Read the model definition and answer for the solid it produces. Units are mm, in the model's axes. A direction names the side the tool comes from. Coordinates: 2 decimals unless noted, no trailing zeros. Order: outer loops, then holes, each group sorted by start corner. A loop starts at its lowest first (then second) coordinate and runs counter-clockwise, first axis right, second up. Notation, with made-up numbers: M -0.5,-21 L 20.5,-21 A11 ccw 20.5,0 Z; hole C 50.25,-29 d5. An arc over 180 degrees is marked long. Write each question's results on one line, items separated by ' | '.
Autodesk Inventor part; units mm, degrees
ref_plane "YZ Plane" through (0, 0, 0) normal (1, 0, 0) x (0, 1, 0)
ref_plane "XZ Plane" through (0, 0, 0) normal (0, 1, 0) x (-1, 0, 0)
ref_plane "XY Plane" through (0, 0, 0) normal (0, 0, 1) x (1, 0, 0)
sketch "Sketch1" plane through (0, 0, 0) normal (0, 0, 1) x (1, 0, 0)
  circle A0 centre (0, 0) radius 1.5
  circle A1 centre (0, 30.5) radius 1.5
  line L0 (0, 8.5) -> (-4, 4.5)
  line L1 (-4, 35) -> (-4, 25.5)
  line L2 (-4, 4.5) -> (-4, -5)
  line L3 (0, 21) -> (0, 8.5)
  line L4 (-4, 35) -> (5, 35)
  line L5 (-4, -5) -> (5, -5)
  line L6 (5, 35) -> (5, -5)
  line L7 (0, 21) -> (0, 23.5)
  line L8 (-4, 25.5) -> (-4, 28)
  line L9 (-4, 28) -> (0, 23.5)
  dimension "d0" = 3
  dimension "d1" = 3
  dimension "d47" = 9
  dimension "d48" = 9
  dimension "d52" = 4
  dimension "d55" = 4.5
  dimension "d59" = 40
  dimension "d60" = 2.5
  dimension "d61" = 2.5
extrude "Extrusion1" add sketch "Sketch1" along normal blind 1
fillet "Fillet9" radius 5 2 edges at (5, 35, 0.5) (5, -5, 0.5)
fillet "Fillet10" radius 4 2 edges at (-4, 35, 0.5) (-4, -5, 0.5)
fillet "Fillet11" radius 7.8 2 edges at (0, 8.5, 0.5) (-4, 4.5, 0.5)
fillet "Fillet12" radius 7.8 2 edges at (-4, 28, 0.5) (0, 23.5, 0.5)
properties part number "arm1" material "ABS Plastic"
(1) Straight lines are drawn through the part: line 1 (X direction, y = 14, z = 0.5); line 2 (X direction, y = 1, z = 0.1); line 3 (Y direction, x = 3, z = 0.75). For each, find the intervals that lie inside material, in ascending order.
Conclusion:
line 1: 0 to 5 | line 2: -4 to -1.12, 1.12 to 5 | line 3: -4 to 34
(2) The part is cut by section D-D, the plane x = 2. Write down the section's boundary in (y, z), then the cut area to 3 significant figures.
Conclusion:
outline: M -4.58,0 L 34.58,0 L 34.58,1 L -4.58,1 Z | area: 39.2 mm²
(3) The mould has two halves that part along X. Classify faces 3 (the cylindrical face through (-1.5, -0.07, 0.49)), 4 (the cylindrical face through (-2.797, 33.859, 0.507)), 5 (the cylindrical face through (3.5, -3.57, 0.51)), 6 (the cylindrical face through (-0.195, 29.013, 0.493)): pulls with the +X half, pulls with the -X half, needs draft (parallel to the pull), parting line crosses it, or undercut.
Conclusion:
face 3: undercut | face 4: pulls with the -X half | face 5: pulls with the +X half | face 6: undercut
(4) The part is cut by section A-A, the plane y = 30.5. Write down the section's boundary in (x, z), then the cut area to 3 significant figures.
Conclusion:
outline: M -3.99,0 L -1.5,0 L -1.5,1 L -3.99,1 Z; M 1.5,0 L 4.97,0 L 4.97,1 L 1.5,1 Z | area: 5.96 mm²
(5) For faces 1 (the cylindrical face through (3.57, 33.5, 0.51)), 2 (the cylindrical face through (-3.505, 28.231, 0.507)), determine the directions among +Z, -Z, +X, -X, +Y, -Y from which every point of the face is accessible in a straight line to the end or side of a thin tool.
Conclusion:
face 1: +Z, -Z, +X, +Y | face 2: +Z, -Z, -X
(6) The part is cut by section C-C, the plane y = 13.5. Write down the section's boundary in (x, z).
Conclusion:
outline: M 0,0 L 5,0 L 5,1 L 0,1 Z
(7) The part is cut by section B-B, the plane z = 0.7. Count the separate pieces of the cut face and the enclosed holes in it, then the cut area to 3 significant figures.
Conclusion:
separate pieces: 1 | enclosed holes: 2 | area: 251 mm²
